Source: CAD feature listing. Evaluate the final solid. Frame: model axes, mm. A direction names the side the tool comes from. Give positions to 0.01 mm unless a question says otherwise; leave off trailing zeros. Write each loop counter-clockwise with the first axis right and the second up, starting at its lowest first coordinate (ties: lowest second). Pieces come first, ordered by that corner, then holes. Notation, with made-up numbers: M -23.75,-24 L -6.75,-24 A23 cw -6.75,-5 Z; hole C -15,40 d7. An arc over 180 degrees is marked long. Return JSON: item names as keys, results as strings.
```python
from build123d import *

# Parameters (mm, degrees)
SKETCH_1_W          = 52
SKETCH_1_H          = 10
EXTRUDE_1_DEPTH     = 1.6
SKETCH_2_R          = 0.8
CUT_EXTRUDE_1_DEPTH = 1.6
SKETCH_3_W          = 14
SKETCH_3_H          = 14
EXTRUDE_3_DEPTH     = 1.6
FILLET_1_R          = 1


with BuildPart() as part:
    # 草图1 → 凸台-拉伸1 (new body)
    with BuildSketch(Plane.XY):
        Rectangle(SKETCH_1_W, SKETCH_1_H)
    extrude(amount=EXTRUDE_1_DEPTH)

    # 草图2 → 切除-拉伸1 (cut)
    with BuildSketch(Plane.XY):
        with Locations((0, 3)):
            Circle(SKETCH_2_R)
        with Locations((0, -3)):
            Circle(SKETCH_2_R)
    extrude(amount=CUT_EXTRUDE_1_DEPTH, mode=Mode.SUBTRACT)

    # 草图3 → 凸台-拉伸3 (add)
    with BuildSketch(Plane.XY):
        with Locations((-19, 0)):
            Rectangle(SKETCH_3_W, SKETCH_3_H)
        with Locations((19, 0)):
            Rectangle(SKETCH_3_W, SKETCH_3_H)
    extrude(amount=EXTRUDE_3_DEPTH)

    # 圆角1
    fillet_1_edges = [part.edges().sort_by_distance(p)[0] for p in [
        (-12, -7, 0.8),
        (-26, 7, 0.8),
        (-26, -7, 0.8),
        (-12, 7, 0.8),
        (12, 7, 0.8),
        (12, -7, 0.8),
        (26, -7, 0.8),
        (26, 7, 0.8),
    ]]
    fillet(fillet_1_edges, radius=FILLET_1_R)


solid = part.part
```
1) Cut plane A-A, the plane z = 0.45. Return the cut outline in (x, y).
Numbers:
{"outline": "M -26,-6 A1 ccw -25,-7 L -13,-7 A1 ccw -12,-6 L -12,-5 L 12,-5 L 12,-6 A1 ccw 13,-7 L 25,-7 A1 ccw 26,-6 L 26,6 A1 ccw 25,7 L 13,7 A1 ccw 12,6 L 12,5 L -12,5 L -12,6 A1 ccw -13,7 L -25,7 A1 ccw -26,6 Z; hole C 0,-3 d1.6; hole C 0,3 d1.6"}
2) Set-up query: faces 5 (the face through (12, 5.5, 0.8)), 6 (the face through (12.301, -6.715, 0.811)), 7 (the face through (-0.17, 2.22, 0.79)). Return all of +Z, -Z, +X, -X, +Y, -Y with unobstructed straight access to the full face (end or side cutting, diameter ignored); none if empty.
Numbers:
{"face 5": "+Z, -Z, +Y", "face 6": "+Z, -Z, -Y", "face 7": "+Z, -Z"}
3) Cut plane C-C, the plane y = 3. Return the cut outline in (x, z), then the cut area to 3 significant figures.
Numbers:
{"outline": "M -26,0 L -0.8,0 L -0.8,1.6 L -26,1.6 Z; M 0.8,0 L 26,0 L 26,1.6 L 0.8,1.6 Z", "area": "80.6 mm²"}
4) Draft query along X for faces 1 (the face through (-25.715, -6.699, 0.811)), 2 (the face through (-12, 5.5, 0.8)), 3 (the face through (25.699, 6.715, 0.811)), 4 (the face through (-12.285, -6.699, 0.811)). Return one class per face: released by +X, released by -X, zero draft, split by the parting line, or undercut.
Numbers:
{"face 1": "released by -X", "face 2": "undercut", "face 3": "released by +X", "face 4": "undercut"}
5) Cut plane B-B, the plane x = 0. Return the cut outline in (y, z), then the cut area to 3 significant figures.
Numbers:
{"outline": "M -5,0 L -3.8,0 L -3.8,1.6 L -5,1.6 Z; M -2.2,0 L 2.2,0 L 2.2,1.6 L -2.2,1.6 Z; M 3.8,0 L 5,0 L 5,1.6 L 3.8,1.6 Z", "area": "10.9 mm²"}
6) Line query: line 1 (Y direction, x = 0, z = 1.25); line 2 (X direction, y = 5.25, z = 0.1); line 3 (Y direction, x = 9, z = 0.6). Output: solid intervals per line, ascending. Write a range as [from, to].
Numbers:
{"line 1": "y = [-5, -3.8], [-2.2, 2.2], [3.8, 5]", "line 2": "x = [-26, -12], [12, 26]", "line 3": "y = [-5, 5]"}
